Geometry check sheet. Reference: the model listing, model coordinates, mm. A direction names the side the tool comes from. Round coordinates to 2 decimals unless told otherwise and drop trailing zeros. Order: outer loops, then holes, each group sorted by start corner. A loop starts at its lowest first (then second) coordinate and runs counter-clockwise, first axis right, second up. Notation, with made-up numbers: (-7.75, 12.25) - (47.25, 12.25) arc R29 ccw to (47.25, 34.25) - close; hole circle Ø2 at (80, 62.5). An arc over 180 degrees is marked (long way). Return JSON: item names as keys, results as strings. Group by question number.
Q1. Sectioned sample at B-B, the plane z = 485. Record the cut outline in (x, y).
Q2. Draft check along X on faces 6 (the flat face through (1935, 43.434, 77)), 7 (the flat face through (2004, 310, 209.55)), 8 (the flat face through (2540, 97, 75)). Enter one of: pulls with the +X half, pulls with the -X half, needs draft (parallel to the pull), parting line crosses it, or undercut.
Q3. Sectioned sample at A-A, the plane y = -47.5. Record the cut outline in (x, z).
Q4. Sectioned sample at D-D, the plane z = 57. Record the cut outline in (x, y), then the cut area to 3 significant figures.
Q5. Material ranges on line 1 along Y through (x, z) = (1762.5, 713.5); line 2 along X through (y, z) = (101, 728.5); line 3 along X through (y, z) = (-482, 54), recorded low to high.
Q6. Tool access check on faces 1 (the flat face through (1841.5, 21, 799)), 2 (the flat face through (1886.98, 273.07, 75.13)), 3 (the flat face through (1994, 124.79, 434)), 4 (the flat face through (1886.98, 273.07, 801.17)), 5 (the flat face through (2290, 0, 75)). Record the directions out of +Z, -Z, +X, -X, +Y, -Y that give a thin tool (end or side, any length) a straight path to the whole face; none if there is none.
Q7. Sectioned sample at C-C, the plane x = 365. Record the cut outline in (y, z), then the cut area to 3 significant figures.
Q8. Gauge pin test, flat ends, axial feed: pin 1 Ø7.5 at (y, z) = (306, 653) entering from +X; pin 2 Ø8 at (y, z) = (180.5, 460.5) entering from -X; pin 3 Ø19 at (x, z) = (2162, 644) entering from -Y; pin 4 Ø12 at (y, z) = (210.5, 450) entering from +X. Record the tip position at first contact, or that the pin passes through.
```python
from build123d import *

# Parameters (mm, degrees)
BOSS_EXTRUDE1_DEPTH  = 152.4
SKETCH2_W            = 190.5
SKETCH2_H            = 190.5
CUT_EXTRUDE1_DEPTH   = 254
BOSS_EXTRUDE2_DEPTH  = 571.5
FILLET1_R            = 127
FILLET1_OF_MIRROR1_R = 127
SKETCH8_W            = 127
SKETCH8_H            = 25.4
BOSS_EXTRUDE3_DEPTH  = 38.1
CUT_EXTRUDE2_DEPTH   = 43.18


with BuildPart() as part:
    # Sketch1 → Boss-Extrude1 (new body)
    with BuildSketch(Plane.XY):
        with BuildLine():
            Line((213.019747539, -692.104923164), (213.019747539, -628.039977762))
            ThreePointArc((213.019747539, -628.039977762), (222.347003261, -589.92262974), (248.221012719, -560.418976506))
            Line((248.221012719, -560.418976506), (1260.898352267, 148.66533042))
            ThreePointArc((1260.898352267, 148.66533042), (1269.688171281, 155.409995769), (1277.856706062, 162.895078834))
            Line((1277.856706062, 162.895078834), (1307.506572341, 192.544945114))
            ThreePointArc((1307.506572341, 192.544945114), (1343.636614311, 217.843472857), (1386.240354223, 229.259110561))
            Line((1386.240354223, 229.259110561), (2540, 330.2))
            Line((2540, 330.2), (2540, 0))
            Line((2540, 0), (1470.214730938, 0))
            ThreePointArc((1470.214730938, 0), (1279.266548253, -29.389736275), (1105.993693855, -114.838451876))
            Line((1105.993693855, -114.838451876), (281.571733527, -692.104923164))
            Line((281.571733527, -692.104923164), (213.019747539, -692.104923164))
        make_face()
    boss_extrude1 = extrude(amount=BOSS_EXTRUDE1_DEPTH)

    # Sketch2 → Cut-Extrude1 (cut)
    with BuildSketch(Plane.XY.offset(152.4)):
        with Locations((1936.75, -51.816)):
            Rectangle(SKETCH2_W, SKETCH2_H)
    cut_extrude1 = extrude(amount=-CUT_EXTRUDE1_DEPTH, mode=Mode.SUBTRACT)

    # Sketch4 → Boss-Extrude2 (add)
    with BuildSketch(Plane.XY.offset(152.4)):
        with BuildLine():
            Line((1581.15, 124.78955528), (2419.35, 124.78955528))
            ThreePointArc((2419.35, 124.78955528), (2437.310512242, 132.229043038), (2444.75, 150.18955528))
            Line((2444.75, 150.18955528), (2444.75, 175.58955528))
            ThreePointArc((2444.75, 175.58955528), (2437.310512242, 193.550067523), (2419.35, 200.98955528))
            Line((2419.35, 200.98955528), (1581.15, 200.98955528))
            ThreePointArc((1581.15, 200.98955528), (1563.189487758, 193.550067523), (1555.75, 175.58955528))
            Line((1555.75, 175.58955528), (1555.75, 150.18955528))
            ThreePointArc((1555.75, 150.18955528), (1563.189487758, 132.229043038), (1581.15, 124.78955528))
        make_face()
    extrude(amount=BOSS_EXTRUDE2_DEPTH)

    # Fillet1
    fillet1_edges = [part.edges().sort_by_distance(p)[0] for p in [
        (2540, 330.2, 76.2),
    ]]
    fillet(fillet1_edges, radius=FILLET1_R)

    # Mirror1: Boss-Extrude1, Cut-Extrude1 across plane
    add(boss_extrude1.mirror(Plane.XY.offset(438.15)))
    add(cut_extrude1.mirror(Plane.XY.offset(438.15)), mode=Mode.SUBTRACT)

    # Fillet1 of Mirror1
    fillet1_of_mirror1_edges = [part.edges().sort_by_distance(p)[0] for p in [
        (2540, 330.2, 800.1),
    ]]
    fillet(fillet1_of_mirror1_edges, radius=FILLET1_OF_MIRROR1_R)

    # Sketch8 → Boss-Extrude3 (add)
    with BuildSketch(Plane.XY.offset(247.65)):
        with BuildLine():
            Line((1708.15, 200.98955528), (1708.15, 378.78955528))
            ThreePointArc((1708.15, 378.78955528), (1719.309231637, 405.730323644), (1746.25, 416.88955528))
            Line((1746.25, 416.88955528), (2254.25, 416.88955528))
            ThreePointArc((2254.25, 416.88955528), (2281.190768363, 405.730323644), (2292.35, 378.78955528))
            Line((2292.35, 378.78955528), (2292.35, 200.98955528))
            Line((2292.35, 200.98955528), (1708.15, 200.98955528))
        make_face()
        with Locations((1835.15, 308.93955528)):
            Rectangle(SKETCH8_W, SKETCH8_H, mode=Mode.SUBTRACT)
        with Locations((2165.35, 308.93955528)):
            Rectangle(SKETCH8_W, SKETCH8_H, mode=Mode.SUBTRACT)
    boss_extrude3 = extrude(amount=-BOSS_EXTRUDE3_DEPTH)

    # Sketch9 → Cut-Extrude2 (cut)
    with BuildSketch(Plane.XY.offset(247.65)):
        with BuildLine():
            Line((1936.75, 385.13955528), (1936.75, 416.88955528))
            Line((1936.75, 416.88955528), (2000.25, 416.88955528))
            Line((2000.25, 416.88955528), (2000.25, 385.13955528))
            ThreePointArc((2000.25, 385.13955528), (1968.5, 353.38955528), (1936.75, 385.13955528))
        make_face()
    cut_extrude2 = extrude(amount=-CUT_EXTRUDE2_DEPTH, mode=Mode.SUBTRACT)

    # Mirror2: Boss-Extrude3, Cut-Extrude2 across plane
    add(boss_extrude3.mirror(Plane.XY.offset(438.15)))
    add(cut_extrude2.mirror(Plane.XY.offset(438.15)), mode=Mode.SUBTRACT)


solid = part.part
```
Reply:
{
 "1": {"outline": "(1555.75, 150.19) arc R25.4 ccw to (1581.15, 124.79) - (2419.35, 124.79) arc R25.4 ccw to (2444.75, 150.19) - (2444.75, 175.59) arc R25.4 ccw to (2419.35, 200.99) - (1581.15, 200.99) arc R25.4 ccw to (1555.75, 175.59) - close"},
 "2": {"face 6": "undercut", "face 7": "needs draft", "face 8": "pulls with the +X half"},
 "3": {"outline": "(980.75, 0) - (1229.24, 0) - (1229.24, 152.4) - (980.75, 152.4) - close; (980.75, 723.9) - (1229.24, 723.9) - (1229.24, 876.3) - (980.75, 876.3) - close"},
 "4": {"outline": "(213.02, -692.1) - (281.57, -692.1) - (1105.99, -114.84) arc R635 cw to (1470.21, 0) - (1841.5, 0) - (1841.5, 43.43) - (2032, 43.43) - (2032, 0) - (2540, 0) - (2540, 191.6) arc R127 ccw to (2401.93, 318.12) - (1386.24, 229.26) arc R127 ccw to (1307.51, 192.54) - (1277.86, 162.9) arc R127 cw to (1260.9, 148.67) - (248.22, -560.42) arc R82.55 ccw to (213.02, -628.04) - close", "area": "500,000 mm^2"},
 "5": {"line 1": "124.79 to 200.99", "line 2": "1192.83 to 2540", "line 3": "360.21 to 581.63"},
 "6": {"face 1": "+Z, -Z, -Y", "face 2": "-Z, -X, +Y", "face 3": "+X, -X, -Y", "face 4": "+Z, -X, +Y", "face 5": "+Z, -Z, +X, -Y"},
 "7": {"outline": "(-633.69, 0) - (-478.65, 0) - (-478.65, 152.4) - (-633.69, 152.4) - close; (-633.69, 723.9) - (-478.65, 723.9) - (-478.65, 876.3) - (-633.69, 876.3) - close", "area": "47,300 mm^2"},
 "8": {"pin 1": "x = 2292.35", "pin 2": "x = 1555.77", "pin 3": "y = 124.79", "pin 4": "through"}
}
